Input: part model. Units: mm. Frame: model coordinates. Give positions to 0.01 mm unless a question says otherwise; leave off trailing zeros. Write each loop counter-clockwise with the first axis right and the second up, starting at its lowest first coordinate (ties: lowest second). Pieces come first, ordered by that corner, then holes. Notation, with made-up numbers: (5.5, 12) - (12.5, 12) arc R20 cw to (12.5, 46) - close; hole circle Ø2 at (-35, 55.25). An arc over 180 degrees is marked (long way). Use a Markdown table: item, result. Add a question column.
1. Section query C-C, the plane z = 0. Return loops of the section in (x, y), plus the area to 3 significant figures.
2. Section query B-B, the plane y = 1.35. Return loops of the section in (x, z).
3. Mould query, pull axis Z, two halves, no side actions, for faces 1 (the flat face through (-12.5, 2, -1)), 2 (the cylindrical face through (-0.62, 2.46, 32.79)), 3 (the cylindrical face through (0, 2, 50)). Classes: released by +Z, released by -Z, zero draft, split by the parting line, or undercut.
4. Pin query (flat end, axial travel): pin 1 (2 mm diameter, centred on x = -3.5, y = 1, fed in from +Z); pin 2 (1 mm diameter, centred on x = 3.5, y = 3, fed in from +Z); pin 3 (1.5 mm diameter, centred on x = -5.5, y = 4, fed in from -Z). Return the tip coordinate at first contact, or that it passes through.
5. Material intervals for probe 1 along X at (y, z) = (2.2, 0); probe 2 along Z at (x, y) = (0, 4.05); probe 3 along Z at (x, y) = (2.5, 4.55), sorted ascending.
6. Section query D-D, the plane x = 6.5. Return loops of the section in (y, z).
7. Section query A-A, the plane x = 0. Return loops of the section in (y, z), plus the area to 3 significant figures.
```python
from build123d import *

# Parameters (mm, degrees)
SKETCH1_R           = 12.5
SKETCH1_R_2         = 4.75
SKETCH1_R_3         = 2.1
BOSS_EXTRUDE1_DEPTH = 5


with BuildPart() as part:
    # Sketch1 → Boss-Extrude1 (new body)
    with BuildSketch(Plane(origin=(0, 0, 0), x_dir=(1, 0, 0), z_dir=(0, 1, 0))):
        with Locations((0, 37.5)):
            Circle(SKETCH1_R)
        with Locations((0, 37.5)):
            Circle(SKETCH1_R_2, mode=Mode.SUBTRACT)
        with BuildLine():
            ThreePointArc((-12.5, -37.5), (0, -25), (12.5, -37.5))
            Line((12.5, -37.5), (12.5, 37.5))
            ThreePointArc((12.5, 37.5), (4.5e-08, 25), (-12.5, 37.49999991))
            Line((-12.5, 37.49999991), (-12.5, -37.5))
        make_face()
        with Locations((-6.5, 0)):
            Circle(SKETCH1_R_3, mode=Mode.SUBTRACT)
        with Locations((6.5, 0)):
            Circle(SKETCH1_R_3, mode=Mode.SUBTRACT)
        with Locations((0, -37.5)):
            Circle(SKETCH1_R)
        with Locations((0, -37.5)):
            Circle(SKETCH1_R_2, mode=Mode.SUBTRACT)
    extrude(amount=BOSS_EXTRUDE1_DEPTH)


solid = part.part
```
Result sheet:
| question | item | result |
|---|---|---|
| 1 | outline | (-12.5, 0) - (-8.6, 0) - (-8.6, 5) - (-12.5, 5) - close; (-4.4, 0) - (4.4, 0) - (4.4, 5) - (-4.4, 5) - close; (8.6, 0) - (12.5, 0) - (12.5, 5) - (8.6, 5) - close |
| 1 | area | 83.0 mm² |
| 2 | outline | (-12.5, -37.5) arc R12.5 ccw to (12.5, -37.5) - (12.5, 37.5) arc R12.5 ccw to (-12.5, 37.5) - close; hole circle Ø4.2 at (-6.5, 0); hole circle Ø9.5 at (0, -37.5); hole circle Ø9.5 at (0, 37.5); hole circle Ø4.2 at (6.5, 0) |
| 3 | face 1 | zero draft |
| 3 | face 2 | undercut |
| 3 | face 3 | released by +Z |
| 4 | pin 1 | stops at z = 49.75 |
| 4 | pin 2 | stops at z = 49.63 |
| 4 | pin 3 | stops at z = -49.06 |
| 5 | probe 1 | x = -12.5 to -8.6, -4.4 to 4.4, 8.6 to 12.5 |
| 5 | probe 2 | z = -50 to -42.25, -32.75 to 32.75, 42.25 to 50 |
| 5 | probe 3 | z = -49.75 to -41.54, -33.46 to 33.46, 41.54 to 49.75 |
| 6 | outline | (0, -48.18) - (5, -48.18) - (5, -2.1) - (0, -2.1) - close; (0, 2.1) - (5, 2.1) - (5, 48.18) - (0, 48.18) - close |
| 7 | outline | (0, -50) - (5, -50) - (5, -42.25) - (0, -42.25) - close; (0, -32.75) - (5, -32.75) - (5, 32.75) - (0, 32.75) - close; (0, 42.25) - (5, 42.25) - (5, 50) - (0, 50) - close |
| 7 | area | 405 mm² |
